The listing builds one solid part. Answer for the finished solid, in the listing's coordinates (mm). A direction names the side the tool comes from. Round coordinates to 2 decimals unless told otherwise and drop trailing zeros. Write each loop counter-clockwise with the first axis right and the second up, starting at its lowest first coordinate (ties: lowest second). Pieces come first, ordered by that corner, then holes.
from build123d import *

# Parameters (mm, degrees)
CROQUIS1_W              = 55
CROQUIS1_H              = 40
SALIENTE_EXTRUIR1_DEPTH = 3
CROQUIS2_W              = 15
CROQUIS2_H              = 6
CORTAR_EXTRUIR1_DEPTH   = 35.528973341
CROQUIS3_R              = 4
CORTAR_EXTRUIR2_DEPTH   = 35.528973341
REDONDEO1_R             = 5


with BuildPart() as part:
    # Croquis1 → Saliente-Extruir1 (new, symmetric)
    with BuildSketch(Plane(origin=(0, 0, 0), x_dir=(1, 0, 0), z_dir=(0, 1, 0))):
        Rectangle(CROQUIS1_W, CROQUIS1_H)
    extrude(amount=SALIENTE_EXTRUIR1_DEPTH, both=True)

    # Croquis2 → Cortar-Extruir1 (cut, through all)
    with BuildSketch(Plane(origin=(0, -3, 0), x_dir=(-1, 0, 0), z_dir=(0, -1, 0))):
        with Locations((17.5, -14)):
            Rectangle(CROQUIS2_W, CROQUIS2_H)
        with Locations((-17.5, -14)):
            Rectangle(CROQUIS2_W, CROQUIS2_H)
        with Locations((17.5, 14)):
            Rectangle(CROQUIS2_W, CROQUIS2_H)
        with Locations((-17.5, 14)):
            Rectangle(CROQUIS2_W, CROQUIS2_H)
    extrude(amount=-CORTAR_EXTRUIR1_DEPTH, mode=Mode.SUBTRACT)

    # Croquis3 → Cortar-Extruir2 (cut, through all)
    with BuildSketch(Plane(origin=(0, -3, 0), x_dir=(-1, 0, 0), z_dir=(0, -1, 0))):
        with Locations(Location((0, 0, 0), (0, 0, 90))):
            Circle(CROQUIS3_R)
    extrude(amount=-CORTAR_EXTRUIR2_DEPTH, mode=Mode.SUBTRACT)

    # Redondeo1
    redondeo1_edges = [part.edges().sort_by_distance(p)[0] for p in [
        (27.5, 0, 20),
        (-27.5, 0, 20),
        (-27.5, 0, -20),
        (27.5, 0, -20),
    ]]
    fillet(redondeo1_edges, radius=REDONDEO1_R)


solid = part.part
1. Section D-D on x = -17 is taken. Determine the outline of the cut face in (y, z), plus the area to 3 significant figures.
Geometry says:
outline: (-3, -20) - (3, -20) - (3, -17) - (-3, -17) - close; (-3, -11) - (3, -11) - (3, 11) - (-3, 11) - close; (-3, 17) - (3, 17) - (3, 20) - (-3, 20) - close
area: 168 mm2
2. Section B-B on z = 0 is taken. Determine the outline of the cut face in (x, y).
Geometry says:
outline: (-27.5, -3) - (-4, -3) - (-4, 3) - (-27.5, 3) - close; (4, -3) - (27.5, -3) - (27.5, 3) - (4, 3) - close
3. Straight lines are drawn through the part: line 1 along Z through (x, y) = (-19.5, -1.65); line 2 along X through (y, z) = (0.05, 0); line 3 along Z through (x, y) = (-23.5, 1.9). For each, find the intervals that lie inside material, in ascending order.
Geometry says:
line 1: z = -20 to -17, -11 to 11, 17 to 20
line 2: x = -27.5 to -4, 4 to 27.5
line 3: z = -19.9 to -17, -11 to 11, 17 to 19.9
4. Section A-A on x = 0 is taken. Determine the outline of the cut face in (y, z).
Geometry says:
outline: (-3, -20) - (3, -20) - (3, -4) - (-3, -4) - close; (-3, 4) - (3, 4) - (3, 20) - (-3, 20) - close
5. For a pull along Z with two mould halves and no side action, classify faces 1 (the face through (0, 0, -20)), 2 (the face through (-27.5, 0, 0)), 3 (the face through (-17, 0, 17)) as released by +Z, released by -Z, zero draft, split by the parting line, or undercut.
Geometry says:
face 1: released by -Z
face 2: zero draft
face 3: undercut
6. Section C-C on y = 0.7 is taken. Determine the outline of the cut face in (x, z), plus the area to 3 significant figures.
Geometry says:
outline: (-27.5, -15) arc R5 ccw to (-22.5, -20) - (22.5, -20) arc R5 ccw to (27.5, -15) - (27.5, 15) arc R5 ccw to (22.5, 20) - (-22.5, 20) arc R5 ccw to (-27.5, 15) - close; hole (-25, -17) - (-10, -17) - (-10, -11) - (-25, -11) - close; hole (-25, 11) - (-10, 11) - (-10, 17) - (-25, 17) - close; hole circle Ø8 at (0, 0); hole (10, -17) - (25, -17) - (25, -11) - (10, -11) - close; hole (10, 11) - (25, 11) - (25, 17) - (10, 17) - close
area: 1,770 mm2
7. A tool of negligible diameter and unlimited length cuts with its end or side. For faces 4 (the face through (18, 0, 17)), 5 (the face through (-26.07, -0.04, -18.5)), from which of +Z, -Z, +X, -X, +Y, -Y can it reach the whole face along a straight path? Write none if from no direction.
Geometry says:
face 4: +Y, -Y
face 5: -Z, -X, +Y, -Y
